Geometry check sheet. Reference: the model listing, model coordinates, mm. A direction names the side the tool comes from. Give positions to 0.01 mm unless a question says otherwise; leave off trailing zeros. Write each loop counter-clockwise with the first axis right and the second up, starting at its lowest first coordinate (ties: lowest second). Pieces come first, ordered by that corner, then holes. Notation, with made-up numbers: (-9.75, 88) - (46.25, 88) arc R9 ccw to (46.25, 92) - close; hole circle Ø6 at (54, 44). An arc over 180 degrees is marked (long way). Use a Markdown table: item, result.
Autodesk Fusion 360 part; units mm, degrees
sketch "Sketch1" plane through (0, 0, 0) normal (0, 0, 1) x (1, 0, 0)
  line L0 (-1.05, 4.05) -> (1.15, 4.05)
  line L1 (1.15, 4.05) -> (1.15, -4.15)
  line L2 (1.15, -4.15) -> (-1.05, -4.15)
  line L3 (-1.05, 0.9) -> (-4, 0.9)
  line L4 (-4, 0.9) -> (-4, -0.8)
  line L5 (-4, -0.8) -> (-1.05, -0.8)
  line L6 (1.15, -0.9) -> (1.15, 0.9)
  line L7 (-1.05, -4.15) -> (-1.05, -0.8)
  line L8 (-1.05, 0.9) -> (-1.05, 4.05)
  dimension "d1" = 2.2
  dimension "d2" = 8.2
  dimension "d4" = 4.15
  dimension "d5" = 1.15
  dimension "d6" = 1.7
  dimension "d7" = 0.9
  dimension "d12" = 4
extrude "Extrude1" add sketch "Sketch1" along normal blind 6.814
equation "d1 = 2.5 mm - 0.3 mm"
equation "d2 = 8.60 mm - 0.4 mm"
equation "d4 = ( 8.3 / 2 ) * 1 mm"
equation "d5 = ( 2.3 / 2 ) * 1 mm"
equation "d6 = 2 mm - 0.3 mm"
equation "d7 = ( 1.8 / 2 ) * 1 mm"
equation "d10 = 6.964 mm - 0.15 mm"
equation "d12 = 4.3 mm - 0.3 mm"
1) Section check A-A on z = 1.75. Record the boundary of the cut face in (x, y), then the cut area to 3 significant figures.
Working result:
| item | result |
|---|---|
| outline | (-4, -0.8) - (-1.05, -0.8) - (-1.05, -4.15) - (1.15, -4.15) - (1.15, 4.05) - (-1.05, 4.05) - (-1.05, 0.9) - (-4, 0.9) - close |
| area | 23.1 mm² |
2) Section check C-C on y = -3.25. Record the boundary of the cut face in (x, z), then the cut area to 3 significant figures.
Working result:
| item | result |
|---|---|
| outline | (-1.05, 0) - (1.15, 0) - (1.15, 6.81) - (-1.05, 6.81) - close |
| area | 15.0 mm² |
3) Section check B-B on x = -3.15. Record the boundary of the cut face in (y, z), then the cut area to 3 significant figures.
Working result:
| item | result |
|---|---|
| outline | (-0.8, 0) - (0.9, 0) - (0.9, 6.81) - (-0.8, 6.81) - close |
| area | 11.6 mm² |
4) Depth check by flat-ended pin: P1, Ø1, axis at y = 2.5, z = 1, coming from the -X side; P2, Ø2.5, axis at x = -3, z = 4, coming from the -Y side; P3, Ø0.9, axis at x = -2, z = 3.5, coming from the +Y side. Enter the tip coordinate at first touch or a pass-through.
Working result:
| item | result |
|---|---|
| P1 | stops at x = -1.05 |
| P2 | stops at y = -0.8 |
| P3 | stops at y = 0.9 |
5) Material ranges on L1, parallel to X at y = -3.5, z = 6.5; L2, parallel to Y at x = -1.8, z = 0.5, recorded low to high. Write a range as from..to.
Working result:
| item | result |
|---|---|
| L1 | x = -1.05..1.15 |
| L2 | y = -0.8..0.9 |
6) Set-up check for faces 1 (the flat face through (0, -4.15, 3)), 2 (the flat face through (-3, -0.8, 3)), 3 (the flat face through (-1.05, 2, 3)): record each of +Z, -Z, +X, -X, +Y, -Y from which the full face is reachable in a straight line by a thin tool's end or side.
Working result:
| item | result |
|---|---|
| face 1 | +Z, -Z, +X, -X, -Y |
| face 2 | +Z, -Z, -X, -Y |
| face 3 | +Z, -Z, -X, +Y |
